from build123d import *

# Parameters (mm, degrees)
F0_W           = 55
F0_H           = 42
F1_DEPTH       = 15
F3_DEPTH       = 8
F4_DEPTH       = 3.1
F4_DEPTH_BACK  = 11
F6_D           = 7
F6_CSINK_D     = 12
F6_CSINK_ANGLE = 90


# Not quite as in the source:
# - a pattern or mirror of a feature is missing from the dataset's text; its kind, count and spacing are read off the source's solid


with BuildPart() as f1:
    # F0 (on Front) → F1 (new body)
    with BuildSketch(Plane.XZ):
        with Locations((0, -21)):
            Rectangle(F0_W, F0_H)
    extrude(amount=-F1_DEPTH)

    # F2 (on face) → F3 (join)
    with BuildSketch(Plane.YZ.offset(27.5)):
        with BuildLine():
            Line((0, -42), (0, -21.960586854))
            Line((0, -21.960586854), (-26.9221419573, -47.7830788612))
            ThreePointArc((-26.9221419573, -47.7830788612), (-16.0770814164, -45.8015919972), (-10, -55))
            ThreePointArc((-10, -55), (-10.8015919972, -58.9229185836), (-13.0778580427, -62.2169211388))
            Line((-13.0778580427, -62.2169211388), (8, -42))
            Line((8, -42), (0, -42))
        make_face()
        with BuildLine():
            ThreePointArc((-10, -55), (-16.0770814164, -45.8015919972), (-26.9221419573, -47.7830788612))
            Line((-26.9221419573, -47.7830788612), (-13.0778580427, -62.2169211388))
            ThreePointArc((-13.0778580427, -62.2169211388), (-10.8015919972, -58.9229185836), (-10, -55))
        make_face()
    f3 = extrude(amount=-F3_DEPTH)

    # F3_copies: F3 across plane
    add(f3.mirror(Plane(origin=(0, 0, 0), x_dir=(0, 0, -1), z_dir=(-1, 0, 0))))

    # F2 (on face) → F4 (join, two sides)
    with BuildSketch(Plane.YZ.offset(27.5)) as f4_sk:
        with BuildLine():
            Line((-13.0778580427, -62.2169211388), (-26.9221419573, -47.7830788612))
            ThreePointArc((-26.9221419573, -47.7830788612), (-27.2169211388, -61.9221419573), (-13.0778580427, -62.2169211388))
        make_face()
        with BuildLine():
            ThreePointArc((-10, -55), (-16.0770814164, -45.8015919972), (-26.9221419573, -47.7830788612))
            Line((-26.9221419573, -47.7830788612), (-13.0778580427, -62.2169211388))
            ThreePointArc((-13.0778580427, -62.2169211388), (-10.8015919972, -58.9229185836), (-10, -55))
        make_face()
    f4 = extrude(amount=F4_DEPTH) + extrude(f4_sk.sketch, amount=-F4_DEPTH_BACK)

    # F4_copies: F4 across plane
    add(f4.mirror(Plane(origin=(0, 0, 0), x_dir=(0, 0, -1), z_dir=(-1, 0, 0))))

    # F6 (through all)
    with Locations(Plane.XZ):
        with Locations((-15, -10), (0, -30)):
            f6 = CounterSinkHole(F6_D / 2, F6_CSINK_D / 2, counter_sink_angle=F6_CSINK_ANGLE)

    # F6_copies: F6 across plane
    add(f6.mirror(Plane(origin=(0, 0, 0), x_dir=(0, 0, 1), z_dir=(1, 0, 0))), mode=Mode.SUBTRACT)


solid = f1.part
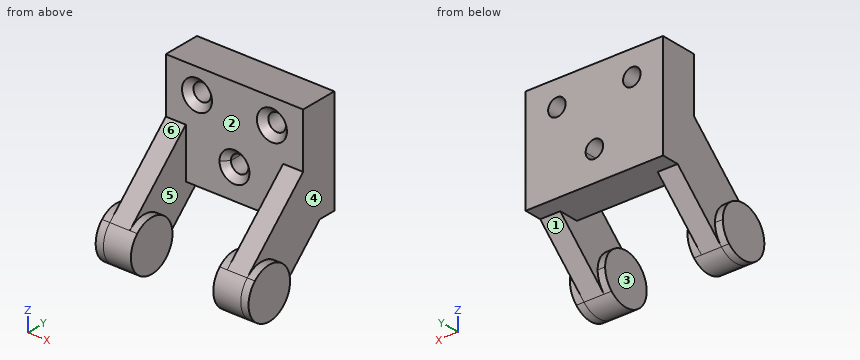
Could you check a few things on this model? Use its own coordinates, in mm. Face numbers are marked on the shaded views. A direction names the side the tool comes from. Give positions to 0.01 mm unless a question says otherwise; leave off trailing zeros. Order: outer loops, then holes, each group sorted by start corner. A loop starts at its lowest first (then second) coordinate and runs counter-clockwise, first axis right, second up.
1. For the marked faces 1, 2 and 3, which set-ups out of +Z, -Z, +X, -X, +Y, -Y let a thin tool reach every point of the face, with its end or its side?
2. Will these pins go through, and if not, where does the flat tip stop? P1, Ø21, axis at x = 5.5, z = -30, coming from the -Y side; P2, Ø8, axis at y = 9, z = -8, coming from the +X side; P3, Ø6, axis at x = 19.5, y = -17, coming from the -Z side; P4, Ø4.5, axis at x = -8.5, y = 8, coming from the -Z side.
3. We'd pull the mould along X, two halves only. Please class the marked faces 4, 5 and 6: pulls with the +X half, pulls with the -X half, needs draft (parallel to the pull), parting line crosses it, or undercut.
4. Suppose I cut it at C-C (z = -10). List the corners of the cut face in (x, y) for me.
5. Suppose I cut it at A-A (y = 10). List the corners of the cut face in (x, z) for me.
6. Suppose I cut it at D-D (y = -23). List the corners of the cut face in (x, z) for me.
7. I need wall thicknesses on L1, parallel to X at y = 6, z = -10; L2, parallel to Z at x = -15, y = 10; L3, parallel to X at y = -13.5, z = -39. Which ranges of each line are inside material? Lowest first, please.
8. Suppose I cut it at B-B (x = -15). List the corners of the cut face in (y, z) for me.
Solved:
1. face 1: -Z, +X, -X, +Y
1. face 2: +Z, -Y
1. face 3: +Z, -Z, +Y, -Y
2. P1: stops at y = 0
2. P2: stops at x = 27.5
2. P3: stops at z = -65
2. P4: stops at z = -42
3. face 4: pulls with the +X half
3. face 5: undercut
3. face 6: needs draft
4. outline: (-27.5, 0) - (-21, 0) - (-18.5, 2.5) - (-18.5, 15) - (-27.5, 15) - close; (-11.5, 2.5) - (-9, 0) - (9, 0) - (11.5, 2.5) - (11.5, 15) - (-11.5, 15) - close; (18.5, 2.5) - (21, 0) - (27.5, 0) - (27.5, 15) - (18.5, 15) - close
5. outline: (-27.5, -42) - (27.5, -42) - (27.5, 0) - (-27.5, 0) - close; hole circle Ø7 at (-15, -10); hole circle Ø7 at (0, -30); hole circle Ø7 at (15, -10)
6. outline: (-30.6, -64.54) - (-16.5, -64.54) - (-16.5, -45.46) - (-19.5, -45.46) - (-19.5, -44.02) - (-27.5, -44.02) - (-27.5, -45.46) - (-30.6, -45.46) - close; (16.5, -64.54) - (30.6, -64.54) - (30.6, -45.46) - (27.5, -45.46) - (27.5, -44.02) - (19.5, -44.02) - (19.5, -45.46) - (16.5, -45.46) - close
7. L1: x = -27.5 to -18.5, -11.5 to 11.5, 18.5 to 27.5
7. L2: z = -42 to -13.5, -6.5 to 0
7. L3: x = -27.5 to -19.5, 19.5 to 27.5
8. outline: (0, -42) - (15, -42) - (15, -13.5) - (2.5, -13.5) - (0, -16) - close; (0, -4) - (2.5, -6.5) - (15, -6.5) - (15, 0) - (0, 0) - close
